Source: CAD feature listing. Evaluate the final solid. Frame: model axes, mm. Round coordinates to 2 decimals unless told otherwise and drop trailing zeros. Write each loop counter-clockwise with the first axis right and the second up, starting at its lowest first coordinate (ties: lowest second). Pieces come first, ordered by that corner, then holes. Notation, with made-up numbers: M -20,24 L 6,24 A32 ccw 6,60 Z; hole C -40,48 d4. An arc over 180 degrees is marked long. Answer in a Markdown table with one row per item. Add a question column.
Item 1: Cut plane C-C on z = 14.3. Return loops of the section in (x, y).
Item 2: Contact query for flat-ended pins moving along their axis: pin 1 (1.5 mm diameter, centred on x = 18.5, y = 72, fed in from -Z); pin 2 (2.5 mm diameter, centred on x = 19.48, y = 43.29, fed in from +Z). Output: stop coordinate, or through.
Item 3: Cut plane A-A on x = 7.25. Return loops of the section in (y, z), and give its area (3 significant figures).
Item 4: Cut plane D-D on x = 12.25. Return loops of the section in (y, z), and give its area (3 significant figures).
Item 5: Cut plane B-B on y = 70.5. Return loops of the section in (x, z), and give its area (3 significant figures).
Item 6: Material intervals for probe 1 along Z at (x, y) = (10.5, 55); probe 2 along Y at (x, z) = (6, 17.2); probe 3 along Y at (x, z) = (21, 17.4), sorted ascending.
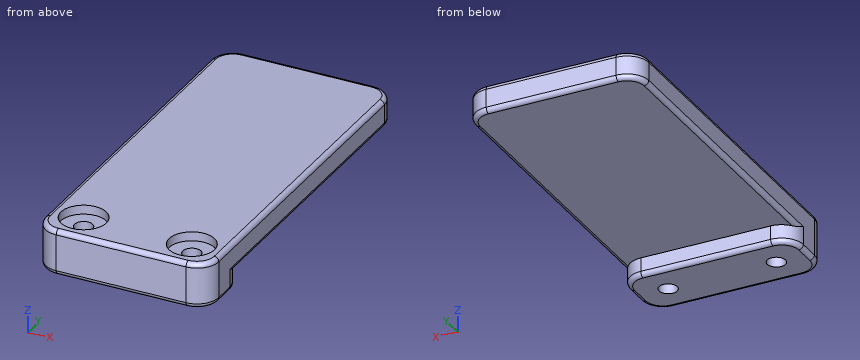
from build123d import *

# Parameters (mm, degrees)
SKETCH007_W     = 19.05
SKETCH007_H     = 40.48125
SKETCH007_R     = 1
PAD002_DEPTH    = 5
SKETCH008_W     = 33.3375
SKETCH008_H     = 2
POCKET006_DEPTH = 19.051
SKETCH009_R     = 2.5
POCKET007_DEPTH = 1
FILLET006_R     = 2.38125
FILLET007_R     = 0.5


with BuildPart() as part:
    # Sketch007 → Pad002 (new body)
    with BuildSketch(Plane.XY):
        with Locations((9.525, 55.959375)):
            Rectangle(SKETCH007_W, SKETCH007_H)
        with Locations((3.571875, 39.290625)):
            Circle(SKETCH007_R, mode=Mode.SUBTRACT)
        with Locations((15.478125, 39.290625)):
            Circle(SKETCH007_R, mode=Mode.SUBTRACT)
    extrude(amount=PAD002_DEPTH)

    # Sketch008 (on Face3 of Pad002) → Pocket006 (cut, through all)
    with BuildSketch(Plane(origin=(0, 0, 0), x_dir=(0, -1, 0), z_dir=(-1, 0, 0))):
        with Locations((-59.53125, 1)):
            Rectangle(SKETCH008_W, SKETCH008_H)
    extrude(amount=-POCKET006_DEPTH, mode=Mode.SUBTRACT)

    # Sketch009 (on Face6 of Pocket006) → Pocket007 (cut)
    with BuildSketch(Plane.XY.offset(5)):
        with Locations((3.571875, 39.290625)):
            Circle(SKETCH009_R)
        with Locations((15.478125, 39.290625)):
            Circle(SKETCH009_R)
    extrude(amount=-POCKET007_DEPTH, mode=Mode.SUBTRACT)

    # Fillet006
    fillet006_edges = [part.edges().sort_by_distance(p)[0] for p in [
        (0, 76.2, 3.5),
        (0, 35.71875, 2.5),
        (19.05, 35.71875, 2.5),
        (19.05, 76.2, 3.5),
        (19.05, 42.8625, 1),
        (0, 42.8625, 1),
    ]]
    fillet(fillet006_edges, radius=FILLET006_R)

    # Fillet007
    fillet007_edges = [part.edges().sort_by_distance(p)[0] for p in [
        (0, 58.340625, 2),
        (9.525, 35.71875, 0),
        (0, 55.959375, 5),
    ]]
    fillet(fillet007_edges, radius=FILLET007_R)


with BuildPart() as part_1:
    # Body002 placement: moved
    add(part.part.moved(Location((4, 4, 13))))


solid = part_1.part
Results below:
| question | item | result |
|---|---|---|
| 1 | outline | M 4,42.1 A2.38 ccw 6.38,39.72 L 20.67,39.72 A2.38 ccw 23.05,42.1 L 23.05,44.48 A2.38 ccw 20.67,46.86 L 6.38,46.86 A2.38 ccw 4,44.48 Z; hole C 7.57,43.29 d2; hole C 19.48,43.29 d2 |
| 2 | pin 1 | z = 15 |
| 2 | pin 2 | z = 17 |
| 3 | outline | M 39.72,13.5 A0.5 ccw 40.22,13 L 42.34,13 L 42.34,17 L 40.81,17 L 40.81,18 L 40.22,18 A0.5 ccw 39.72,17.5 Z; M 44.24,13 L 46.36,13 A0.5 ccw 46.86,13.5 L 46.86,15 L 79.7,15 A0.5 ccw 80.2,15.5 L 80.2,17.5 A0.5 ccw 79.7,18 L 45.77,18 L 45.77,17 L 44.24,17 Z |
| 3 | area | 123 mm2 |
| 4 | outline | M 39.72,13.5 A0.5 ccw 40.22,13 L 46.36,13 A0.5 ccw 46.86,13.5 L 46.86,15 L 79.7,15 A0.5 ccw 80.2,15.5 L 80.2,17.5 A0.5 ccw 79.7,18 L 40.22,18 A0.5 ccw 39.72,17.5 Z |
| 4 | area | 135 mm2 |
| 5 | outline | M 4,15.5 A0.5 ccw 4.5,15 L 22.55,15 A0.5 ccw 23.05,15.5 L 23.05,17.5 A0.5 ccw 22.55,18 L 4.5,18 A0.5 ccw 4,17.5 Z |
| 5 | area | 56.9 mm2 |
| 6 | probe 1 | 15 to 18 |
| 6 | probe 2 | 39.75 to 41.35, 45.23 to 80.17 |
| 6 | probe 3 | 39.74 to 41.31, 45.27 to 80.18 |
